```python
from build123d import *

# Parameters (mm, degrees)
SK_BODY_R                = 16
EX_BODY_DEPTH            = 8
SK_BORE_R                = 3
CUT_BORE_DEPTH           = 8
SK_PATTERN16_4XM4_R      = 1.65
CUT_PATTERN16_4XM4_DEPTH = 6


with BuildPart() as part:
    # SK_Body → EX_Body (new body)
    with BuildSketch(Plane(origin=(0, 0, 0), x_dir=(0, 0, -1), z_dir=(1, 0, 0))):
        Circle(SK_BODY_R)
    extrude(amount=EX_BODY_DEPTH)

    # SK_Bore → CUT_Bore (cut)
    with BuildSketch(Plane(origin=(0, 0, 0), x_dir=(0, 0, -1), z_dir=(1, 0, 0))):
        Circle(SK_BORE_R)
    extrude(amount=CUT_BORE_DEPTH, mode=Mode.SUBTRACT)

    # SK_Pattern16_4xM4 → CUT_Pattern16_4xM4 (cut)
    with BuildSketch(Plane(origin=(8, 0, 0), x_dir=(0, 0, -1), z_dir=(1, 0, 0))):
        with Locations((-8, 8)):
            Circle(SK_PATTERN16_4XM4_R)
        with Locations((-8, -8)):
            Circle(SK_PATTERN16_4XM4_R)
        with Locations((8, 8)):
            Circle(SK_PATTERN16_4XM4_R)
        with Locations((8, -8)):
            Circle(SK_PATTERN16_4XM4_R)
    extrude(amount=-CUT_PATTERN16_4XM4_DEPTH, mode=Mode.SUBTRACT)


solid = part.part
```
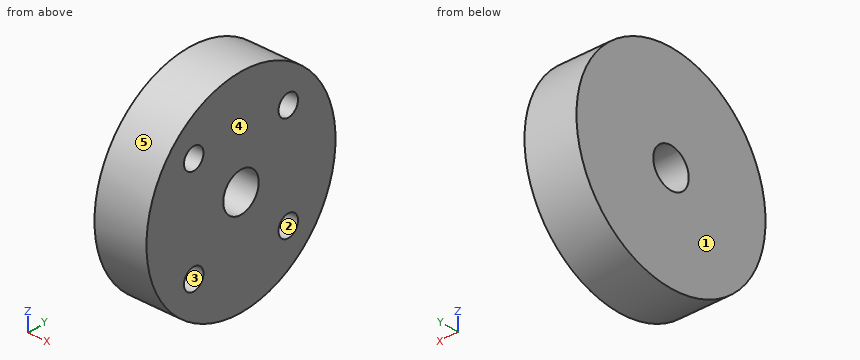
Verification items for the finished model (mm, model axes). Face numbers are marked on the shaded views. A direction names the side the tool comes from. Coordinates: 2 decimals unless noted, no trailing zeros. Write each loop counter-clockwise with the first axis right and the second up, starting at its lowest first coordinate (ties: lowest second). Pieces come first, ordered by that corner, then holes. Notation, with made-up numbers: (34.5, -27.5) - (80.5, -27.5) arc R19 ccw to (80.5, -17.5) - close; hole circle Ø7 at (88.25, 18). An arc over 180 degrees is marked (long way). Write item = value, one per line.
Q1. Go/stop test with flat-tipped pins: pin 1 Ø2 at (x, z) = (5.5, -12.5) entering from -Y; pin 2 Ø2 at (x, z) = (6.5, -7.5) entering from -Y; pin 3 Ø3 at (y, z) = (-8, -8) entering from +X; pin 4 Ø3.5 at (y, z) = (0, 0) entering from -X. Record where each tip stops, or that it passes through.
Answer:
pin_1 = -11.12
pin_2 = -14.62
pin_3 = 2
pin_4 = through
Q2. Material ranges on L1, parallel to Y at x = 7.5, z = -7; L2, parallel to Z at x = 6.5, y = 9; L3, parallel to Y at x = 5.9, z = -8, recorded low to high. Write a range as from..to.
Answer:
L1 = -14.39..-9.31, -6.69..6.69, 9.31..14.39
L2 = -13.23..-9.31, -6.69..6.69, 9.31..13.23
L3 = -13.86..-9.65, -6.35..6.35, 9.65..13.86
Q3. Access from +Z, -Z, +X, -X, +Y, -Y to the whole of each face (thin tool, end or side, straight path). Record for the marked faces 1 and 2.
Answer:
face_1 = +Z, -Z, -X, +Y, -Y
face_2 = +X
Q4. Cross-section at D-D (z = -7.5). Enter the section's corners in (x, y).
Answer:
outline = (0, -14.13) - (8, -14.13) - (8, -9.57) - (2, -9.57) - (2, -6.43) - (8, -6.43) - (8, 6.43) - (2, 6.43) - (2, 9.57) - (8, 9.57) - (8, 14.13) - (0, 14.13) - close
Q5. Cross-section at A-A (y = 0). Enter the section's corners in (x, z).
Answer:
outline = (0, -16) - (8, -16) - (8, -3) - (0, -3) - close; (0, 3) - (8, 3) - (8, 16) - (0, 16) - close
Q6. Cross-section at B-B (x = 3). Enter the section's corners in (y, z).
Answer:
outline = circle Ø32 at (0, 0); hole circle Ø3.3 at (-8, -8); hole circle Ø3.3 at (-8, 8); hole circle Ø6 at (0, 0); hole circle Ø3.3 at (8, -8); hole circle Ø3.3 at (8, 8)
Q7. Mould release check, pull along Z, two halves, no side actions. Record for the marked faces 3, 4 and 5: released by +Z, released by -Z, zero draft, split by the parting line, or undercut.
Answer:
face_3 = undercut
face_4 = zero draft
face_5 = split by the parting line
